Autodesk Inventor part; units mm, degrees
ref_plane "YZ Plane" through (0, 0, 0) normal (1, 0, 0) x (0, 1, 0)
ref_plane "XZ Plane" through (0, 0, 0) normal (0, 1, 0) x (-1, 0, 0)
ref_plane "XY Plane" through (0, 0, 0) normal (0, 0, 1) x (1, 0, 0)
sketch "Sketch1" plane through (0, 0, 0) normal (0, 0, 1) x (1, 0, 0)
  line L0 (0, 0) -> (993, 0)
  line L1 (993, 0) -> (993, 40)
  line L2 (993, 40) -> (0, 40)
  line L3 (0, 40) -> (0, 0)
  dimension "d0" = 993
  dimension "d1" = 40
extrude "Extrusion1" add sketch "Sketch1" along normal blind 10
sketch "Sketch5" plane through (0, 0, 10) normal (0, 0, 1) x (1, 0, 0)
  line L0 (0, 40) -> (0, 0)
  line L1 (0, 20) -> (20.0002, 40)
  line L2 (993, 40) -> (0, 40)
  line L3 (993, 0) -> (993, 40)
  line L4 (993, 20) -> (973.0002, 40)
extrude "Extrusion5" cut sketch "Sketch5" against normal blind 10
properties part number "vslot hinge brace top"
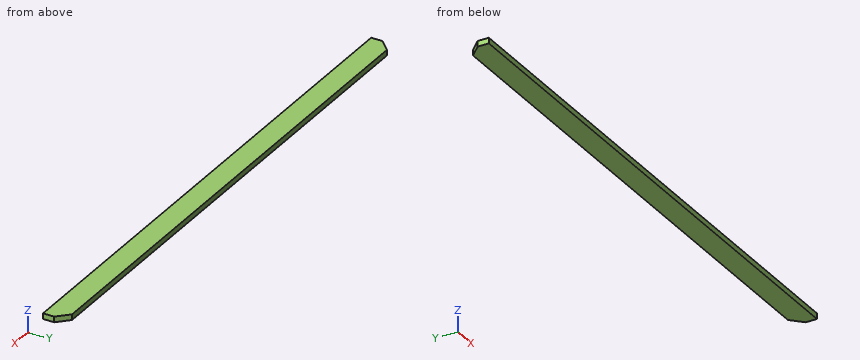
Check sheet for the modelled part. Datum: model origin and axes. Units: mm. Round coordinates to 2 decimals unless told otherwise and drop trailing zeros. Order: outer loops, then holes, each group sorted by start corner. A loop starts at its lowest first (then second) coordinate and runs counter-clockwise, first axis right, second up. Notation, with made-up numbers: (32.5, 78.5) -> (50.5, 78.5) arc R29 ccw to (50.5, 110.5) -> close; hole circle Ø11 at (47.25, 28). An arc over 180 degrees is marked (long way). One line per item, written item: value. Start each with the question number.
Q1. Cross-section at A-A (y = 30). Record the boundary of the cut face in (x, z), and give its area (3 significant figures).
Q2. Thickness scan on line 1 (X direction, y = 36, z = 9); line 2 (X direction, y = 30.5, z = 4.75). Record the ranges inside material, lowest first.
Q3. Gauge pin test, flat end, axial feed: pin 1 Ø4 at (y, z) = (22.5, 4.5) entering from +X. Record the tip position at first contact, or that the pin passes through.
Completed:
1. outline: (10, 0) -> (983, 0) -> (983, 10) -> (10, 10) -> close
1. area: 9,730 mm²
2. line 1: x = 16 to 977
2. line 2: x = 10.5 to 982.5
3. pin 1: stops at x = 992.5
